The listing builds one solid part. Answer for the finished solid, in the listing's coordinates (mm). A direction names the side the tool comes from. Give positions to 0.01 mm unless a question says otherwise; leave off trailing zeros. Order: outer loops, then holes, each group sorted by start corner. A loop starts at its lowest first (then second) coordinate and runs counter-clockwise, first axis right, second up.
```python
from build123d import *

# Parameters (mm, degrees)
DODANIE_WYCI_GNI_CIE1_DEPTH = 1
SZKIC2_W                    = 10
SZKIC2_H                    = 345
DODANIE_WYCI_GNI_CIE2_DEPTH = 2


with BuildPart() as part:
    # Szkic1 → Dodanie-wyciągnięcie1 (new body)
    with BuildSketch(Plane.XY):
        with BuildLine():
            Line((-286.27862804, 196), (-599.968042624, 196))
            Line((-599.968042624, 196), (-599.968042624, 172.5))
            Line((-599.968042624, 172.5), (-649.968042624, 172.5))
            Line((-649.968042624, 172.5), (-649.968042624, -172.5))
            Line((-649.968042624, -172.5), (-599.968042624, -172.5))
            Line((-599.968042624, -172.5), (-599.968042624, -197.196347915))
            Line((-599.968042624, -197.196347915), (-285.747034082, -197.196347915))
            ThreePointArc((-285.747034082, -197.196347915), (-293.157074923, -182.055397704), (-280, -171.517444485))
            Line((-280, -171.517444485), (-280, 172.334252092))
            ThreePointArc((-280, 172.334252092), (-292.242230129, 181.752081969), (-286.27862804, 196))
        make_face()
    extrude(amount=DODANIE_WYCI_GNI_CIE1_DEPTH)

    # Szkic2 → Dodanie-wyciągnięcie2 (add)
    with BuildSketch(Plane(origin=(0, 0, 0), x_dir=(-1, 0, 0), z_dir=(0, 0, -1))):
        with Locations((654.968042624, 0)):
            Rectangle(SZKIC2_W, SZKIC2_H)
    extrude(amount=-DODANIE_WYCI_GNI_CIE2_DEPTH)


solid = part.part
```
1) Find section A-A (z = 0.35). Write down the section's boundary in (x, y), then the cut area to 3 significant figures.
Geometry says:
outline: (-659.97, -172.5) - (-599.97, -172.5) - (-599.97, -197.2) - (-285.75, -197.2) arc R13.48 cw to (-280, -171.52) - (-280, 172.33) arc R12.67 cw to (-286.28, 196) - (-599.97, 196) - (-599.97, 172.5) - (-659.97, 172.5) - close
area: 146,000 mm2
2) For a pull along Y with two mould halves and no side action, classify faces 3 (the cylindrical face through (-292.18, 181.53, 0.49)), 4 (the cylindrical face through (-293.21, -182.3, 0.49)), 5 (the flat face through (-655, 2, 2)) as +Y half, -Y half, draft (parallel to the pull), parting line (faces both ways), or undercut.
Geometry says:
face 3: undercut
face 4: undercut
face 5: draft
3) A tool of negligible diameter and unlimited length cuts with its end or side. For faces 1 (the flat face through (-467, 2, 0)), 2 (the flat face through (-468, 2, 1)), from which of +Z, -Z, +X, -X, +Y, -Y can it reach the whole face along a straight path? Write none if from no direction.
Geometry says:
face 1: -Z, +X, -X, +Y, -Y
face 2: +Z, +X, +Y, -Y
4) Find section B-B (y = 142). Write down the section's boundary in (x, z).
Geometry says:
outline: (-659.97, 0) - (-280, 0) - (-280, 1) - (-649.97, 1) - (-649.97, 2) - (-659.97, 2) - close
5) Find section C-C (x = -584.5). Write down the section's boundary in (y, z), then the cut area to 3 significant figures.
Geometry says:
outline: (-197.2, 0) - (196, 0) - (196, 1) - (-197.2, 1) - close
area: 393 mm2
6) Straight lines are drawn through the part: probe 1 along Z at (x, y) = (-578, 41); probe 2 along X at (y, z) = (-156.5, 1.2); probe 3 along X at (y, z) = (177.5, 0.85). For each, find the intervals that lie inside material, in ascending order.
Geometry says:
probe 1: z = 0 to 1
probe 2: x = -659.97 to -649.97
probe 3: x = -599.97 to -290.21
7) Given P1, Ø10, axis at x = -485.5, y = -123, coming from the +Z side; P2, Ø0.5, axis at y = -188.5, z = 0.5, coming from the -X side; P3, Ø0.5, axis at y = -82, z = 1.5, coming from the +X side, each flat-ended and moving along its own axis, determine where each tip first touches the part or whether it passes through.
Geometry says:
P1: stops at z = 1
P2: stops at x = -599.97
P3: stops at x = -649.97
8) Find section D-D (x = -627). Write down the section's boundary in (y, z).
Geometry says:
outline: (-172.5, 0) - (172.5, 0) - (172.5, 1) - (-172.5, 1) - close
